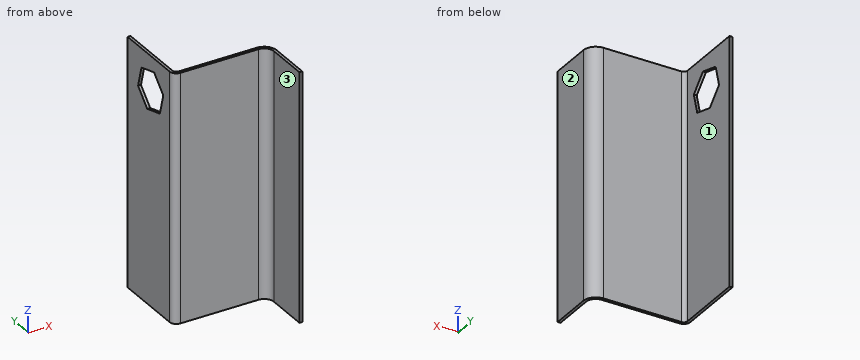
```python
from build123d import *

# Parameters (mm, degrees)
BASE_FLANGE1_DEPTH           = 257.539224292
CUT_EXTRUDE1_DEPTH           = 10
EDGE_FLANGE1_STRIP_W         = 32
EDGE_FLANGE1_STRIP_H         = 3
EDGE_FLANGE1_STRIP_CUT_DEPTH = 257.539224292
EDGE_FLANGE1_DEPTH           = 257.539224292


# Sheet-metal steps are written as plain solids
with BuildPart() as part:
    # Sketch1 → Base-Flange1 (new body)
    with BuildSketch(Plane.XY):
        with BuildLine():
            Line((-53.840389348, 45.270638794), (-53.840389348, -26.739322638))
            ThreePointArc((-53.840389348, -26.739322638), (-52.668816472, -29.567749763), (-49.840389348, -30.739322638))
            Line((-49.840389348, -30.739322638), (44.339144169, -30.739322638))
            Line((44.339144169, -30.739322638), (44.339144169, -33.739322638))
            Line((44.339144169, -33.739322638), (-49.840389348, -33.739322638))
            ThreePointArc((-49.840389348, -33.739322638), (-54.790136816, -31.689070106), (-56.840389348, -26.739322638))
            Line((-56.840389348, -26.739322638), (-56.840389348, 45.270638794))
            Line((-56.840389348, 45.270638794), (-53.840389348, 45.270638794))
        make_face()
    extrude(amount=BASE_FLANGE1_DEPTH)

    # Sketch8 → Cut-Extrude1 (cut)
    with BuildSketch(Plane(origin=(-53.840389348, 0, 0), x_dir=(0, 0, -1), z_dir=(1, 0, 0))):
        Polygon((-216.16259768, 27.390589149), (-237.787839878, 21.496921555), (-243.496395119, -0.177921348), (-227.579708162, -15.959096657), (-205.954465965, -10.065429063), (-200.245910723, 11.60941384), align=None)
    extrude(amount=-CUT_EXTRUDE1_DEPTH, mode=Mode.SUBTRACT)

    # Edge-Flange1 strip (across the edge) → Edge-Flange1 strip cut (cut)
    with BuildSketch(Plane(origin=(44.339144169, -33.739322638, 0), x_dir=(-1, 0, 0), z_dir=(0, 0, 1))):
        with Locations((-3, -1.5)):
            Rectangle(EDGE_FLANGE1_STRIP_W, EDGE_FLANGE1_STRIP_H)
    extrude(amount=EDGE_FLANGE1_STRIP_CUT_DEPTH, mode=Mode.SUBTRACT)

    # Edge-Flange1 section (across the edge) → Edge-Flange1 (add)
    with BuildSketch(Plane(origin=(44.339144169, -33.739322638, 0), x_dir=(-1, 0, 0), z_dir=(0, 0, 1))):
        with BuildLine():
            Line((0, 10), (0, 54))
            Line((0, 54), (3, 54))
            Line((3, 54), (3, 10))
            ThreePointArc((3, 10), (5.928932188, 2.928932188), (13, 0))
            Line((13, 0), (13, -3))
            ThreePointArc((13, -3), (3.807611845, 0.807611845), (0, 10))
        make_face()
    extrude(amount=EDGE_FLANGE1_DEPTH)


solid = part.part
```
Check sheet for the modelled part. Datum: model origin and axes. Units: mm. Face numbers are marked on the shaded views. A direction names the side the tool comes from. Give positions to 0.01 mm unless a question says otherwise; leave off trailing zeros. Order: outer loops, then holes, each group sorted by start corner. A loop starts at its lowest first (then second) coordinate and runs counter-clockwise, first axis right, second up. Notation, with made-up numbers: (64.25, -19) -> (94.25, -19) arc R21 ccw to (94.25, 14) -> close; hole circle Ø7 at (81.25, -36). An arc over 180 degrees is marked (long way). Return JSON: item names as keys, results as strings.
1. Cross-section at C-C, the plane z = 143. Record the cut outline in (x, y), plus the area to 3 significant figures.
From the geometry:
{"outline": "(-56.84, -26.74) arc R7 ccw to (-49.84, -33.74) -> (31.34, -33.74) arc R10 cw to (41.34, -43.74) -> (41.34, -87.74) -> (44.34, -87.74) -> (44.34, -43.74) arc R13 ccw to (31.34, -30.74) -> (-49.84, -30.74) arc R4 cw to (-53.84, -26.74) -> (-53.84, 45.27) -> (-56.84, 45.27) -> close", "area": "672 mm^2"}
2. Set-up check for the marked faces 1, 2 and 3: record each of +Z, -Z, +X, -X, +Y, -Y from which the full face is reachable in a straight line by a thin tool's end or side.
From the geometry:
{"face 1": "+Z, -Z, +X, +Y", "face 2": "+Z, -Z, +X, +Y, -Y", "face 3": "+Z, -Z, -X, -Y"}
3. Cross-section at B-B, the plane y = 6.5. Record the cut outline in (x, z).
From the geometry:
{"outline": "(-56.84, 0) -> (-53.84, 0) -> (-53.84, 201.59) -> (-56.84, 201.59) -> close; (-56.84, 241.74) -> (-53.84, 241.74) -> (-53.84, 257.54) -> (-56.84, 257.54) -> close"}
4. Cross-section at A-A, the plane z = 233. Record the cut outline in (x, y), plus the area to 3 significant figures.
From the geometry:
{"outline": "(-56.84, -26.74) arc R7 ccw to (-49.84, -33.74) -> (31.34, -33.74) arc R10 cw to (41.34, -43.74) -> (41.34, -87.74) -> (44.34, -87.74) -> (44.34, -43.74) arc R13 ccw to (31.34, -30.74) -> (-49.84, -30.74) arc R4 cw to (-53.84, -26.74) -> (-53.84, -10.58) -> (-56.84, -10.58) -> close; (-56.84, 22.8) -> (-53.84, 22.8) -> (-53.84, 45.27) -> (-56.84, 45.27) -> close", "area": "572 mm^2"}
5. Cross-section at D-D, the plane x = 0.5. Record the cut outline in (y, z).
From the geometry:
{"outline": "(-33.74, 0) -> (-30.74, 0) -> (-30.74, 257.54) -> (-33.74, 257.54) -> close"}
6. Material ranges on probe 1 along Y at (x, z) = (22, 70); probe 2 along X at (y, z) = (14, 117.5); probe 3 along X at (y, z) = (-48, 186.5), recorded low to high. Write a range as [from, to].
From the geometry:
{"probe 1": "[-33.74, -30.74]", "probe 2": "[-56.84, -53.84]", "probe 3": "[41.34, 44.34]"}
7. Go/stop test with flat-tipped pins: P1, Ø1, axis at y = 5, z = 191, coming from the +X side; P2, Ø22, axis at y = -57.5, z = 119.5, coming from the -X side; P3, Ø1, axis at x = -2, z = 81.5, coming from the -Y side. Record where each tip stops, or that it passes through.
From the geometry:
{"P1": "x = -53.84", "P2": "x = 41.34", "P3": "y = -33.74"}
